```python
from build123d import *

# Parameters (mm, degrees)
F0_W   = 3
F0_H   = 32
F0_H_2 = 1


with BuildPart() as f1:
    # F0 (on Front) → F1 (revolve)
    with BuildSketch(Plane.XZ):
        with Locations((-1.5, 0)):
            Rectangle(F0_W, F0_H)
        Polygon((-5, 16), (-3, 16), (0, 16), (0, 18.5), (-3, 18.5), (-5, 18.5), align=None)
        Polygon((0, -16), (-3, -16), (-5, -16), (-5, -18.5), (0, -18.5), align=None)
        with Locations((-1.5, 19)):
            Rectangle(F0_W, F0_H_2)
    revolve(axis=Axis((0, 0, 0.5), (0, 0, -1)))


solid = f1.part
```
The listing builds one solid part. Answer for the finished solid, in the listing's coordinates (mm). A direction names the side the tool comes from. Round coordinates to 2 decimals unless told otherwise and drop trailing zeros. Loops run counter-clockwise (first coordinate to the right, second up) from the corner with the lowest first, then second, coordinate; pieces in that order, holes last.
Q1. Find the intervals of material crossed by line 1 (Z direction, x = -1.5, y = 4); line 2 (Y direction, x = 0, z = -6); line 3 (X direction, y = -2.25, z = -9.5), in increasing order.
Q2. For a pull along Z with two mould halves and no side action, classify faces 1 (the face through (0, 0, -18.5)), 2 (the face through (3.3, 0.1, -16)), 3 (the face through (3, 0, 19)), 4 (the face through (3, 0, 0)) as released by +Z, released by -Z, zero draft, split by the parting line, or undercut.
Q3. Given pin 1 Ø1 at (y, z) = (-0.5, -4.5) entering from -X; pin 2 Ø5 at (x, z) = (2.5, 14) entering from -Y, each flat-ended and moving along its own axis, determine where each tip first touches the part or whether it passes through.
Q4. Which of the six approach directions +Z, -Z, +X, -X, +Y, -Y give full straight-line access (tool end or side, diameter ignored) to faces 5 (the face through (1.08, -4.88, 17.23)), 6 (the face through (3.3, 0.1, 18.5)), 7 (the face through (-3.3, 0.1, 16))?
Q5. Section C-C, the plane x = 0 is taken. Determine the outline of the cut face in (y, z), then the cut area to 3 significant figures.
Q6. Section A-A, the plane y = 4 is taken. Determine the outline of the cut face in (x, z).
Completed:
1. line 1: z = -18.5 to -16, 16 to 18.5
1. line 2: y = -3 to 3
1. line 3: x = -1.98 to 1.98
2. face 1: released by -Z
2. face 2: undercut
2. face 3: zero draft
2. face 4: undercut
3. pin 1: stops at x = -3
3. pin 2: stops at y = -4.9
4. face 5: +Z, -Z
4. face 6: +Z
4. face 7: none
5. outline: (-5, -18.5) - (5, -18.5) - (5, -16) - (3, -16) - (3, 16) - (5, 16) - (5, 18.5) - (3, 18.5) - (3, 19.5) - (-3, 19.5) - (-3, 18.5) - (-5, 18.5) - (-5, 16) - (-3, 16) - (-3, -16) - (-5, -16) - close
5. area: 248 mm2
6. outline: (-3, -18.5) - (3, -18.5) - (3, -16) - (-3, -16) - close; (-3, 16) - (3, 16) - (3, 18.5) - (-3, 18.5) - close
